```python
from build123d import *

# Parameters (mm, degrees)
SKETCH1_W           = 7
SKETCH1_H           = 2
BOSS_EXTRUDE1_DEPTH = 33
CUT_EXTRUDE1_REACH  = 35.793
SKETCH2_R           = 2


with BuildPart() as part:
    # Sketch1 → Boss-Extrude1 (new body)
    with BuildSketch(Plane.XY):
        with Locations((3.5, 1)):
            Rectangle(SKETCH1_W, SKETCH1_H)
    extrude(amount=BOSS_EXTRUDE1_DEPTH)

    # Sketch2 → Cut-Extrude1 (cut, up to next)
    with BuildSketch(Plane(origin=(0, 2, 0), x_dir=(1, 0, 0), z_dir=(0, 1, 0)), mode=Mode.PRIVATE) as cut_extrude1_sk1:
        with Locations(Location((3.5, -30, 0), (0, 0, 270))):
            Circle(SKETCH2_R)
    cut_extrude1_tool1 = extrude(cut_extrude1_sk1.sketch, amount=-CUT_EXTRUDE1_REACH, mode=Mode.PRIVATE) & part.part
    # Sketch2 → Cut-Extrude1 (cut, up to next)
    with BuildSketch(Plane(origin=(0, 2, 0), x_dir=(1, 0, 0), z_dir=(0, 1, 0)), mode=Mode.PRIVATE) as cut_extrude1_sk2:
        with Locations(Location((3.5, -3, 0), (0, 0, 270))):
            Circle(SKETCH2_R)
    cut_extrude1_tool2 = extrude(cut_extrude1_sk2.sketch, amount=-CUT_EXTRUDE1_REACH, mode=Mode.PRIVATE) & part.part
    add(cut_extrude1_tool1.solids().sort_by_distance((3.5, 2, 30))[0], mode=Mode.SUBTRACT)
    add(cut_extrude1_tool2.solids().sort_by_distance((3.5, 2, 3))[0], mode=Mode.SUBTRACT)


solid = part.part
```
Source: CAD feature listing. Evaluate the final solid. Frame: model axes, mm. Give positions to 0.01 mm unless a question says otherwise; leave off trailing zeros. Loops run counter-clockwise (first coordinate to the right, second up) from the corner with the lowest first, then second, coordinate; pieces in that order, holes last. Notation, with made-up numbers: (84.5, 33.5) - (131.5, 33.5) arc R15 cw to (131.5, 54.5) - close; hole circle Ø3 at (-29, 86). An arc over 180 degrees is marked (long way). Use CSV: the item, a comma, the result in double quotes.
1) Cut plane D-D (x = 2.25). Output: boundary loops of the cut face in (y, z).
Worked out:
outline,"(0, 0) - (2, 0) - (2, 1.44) - (0, 1.44) - close; (0, 4.56) - (2, 4.56) - (2, 28.44) - (0, 28.44) - close; (0, 31.56) - (2, 31.56) - (2, 33) - (0, 33) - close"
2) Cut plane C-C (y = 1.2). Output: boundary loops of the cut face in (x, z).
Worked out:
outline,"(0, 0) - (7, 0) - (7, 33) - (0, 33) - close; hole circle Ø4 at (3.5, 3); hole circle Ø4 at (3.5, 30)"
3) Line query: line 1 (X direction, y = 1.65, z = 3); line 2 (Z direction, x = 2.25, y = 1.6); line 3 (Z direction, x = 3.25, y = 1.45). Output: solid intervals per line, ascending.
Worked out:
line 1,"x = 0 to 1.5, 5.5 to 7"
line 2,"z = 0 to 1.44, 4.56 to 28.44, 31.56 to 33"
line 3,"z = 0 to 1.02, 4.98 to 28.02, 31.98 to 33"
4) Mould query, pull axis X, two halves, no side actions, for faces 1 (the flat face through (7, 1, 16)), 2 (the cylindrical face through (4.101, 1.014, 4.908)), 3 (the flat face through (3, 2, 16)), 4 (the cylindrical face through (4.101, 1.014, 31.908)). Classes: +X half, -X half, draft (parallel to the pull), parting line (faces both ways), or undercut.
Worked out:
face 1,"+X half"
face 2,"undercut"
face 3,"draft"
face 4,"undercut"
5) Cut plane A-A (z = 3). Output: boundary loops of the cut face in (x, y), and give its area (3 significant figures).
Worked out:
outline,"(0, 0) - (1.5, 0) - (1.5, 2) - (0, 2) - close; (5.5, 0) - (7, 0) - (7, 2) - (5.5, 2) - close"
area,"6.00 mm^2"
6) Cut plane B-B (x = 3.5). Output: boundary loops of the cut face in (y, z), and give its area (3 significant figures).
Worked out:
outline,"(0, 0) - (2, 0) - (2, 1) - (0, 1) - close; (0, 5) - (2, 5) - (2, 28) - (0, 28) - close; (0, 32) - (2, 32) - (2, 33) - (0, 33) - close"
area,"50.0 mm^2"
